Here's the drawing with two shaded views (mm, measured from the low corner). I have some questions. Give positions to 0.01 mm unless a question says otherwise; leave off trailing zeros. Write each loop counter-clockwise with the first axis right and the second up, starting at its lowest first coordinate (ties: lowest second). Pieces come first, ordered by that corner, then holes. Notation, with made-up numbers: M 75,89.5 L 128,89.5 A28 ccw 128,117.5 Z; hole C 43,-32 d9. An arc over 180 degrees is marked long. Answer as CSV lines item,"result". Start each with the question number.
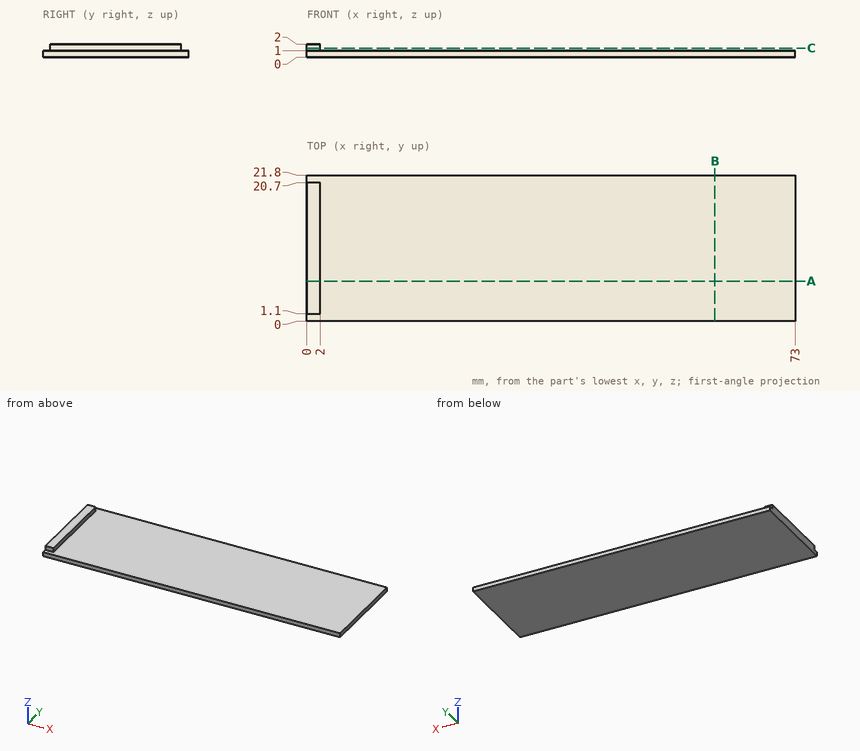
1. Will these pins go through, and if not, where does the flat tip stop? P1, Ø0.8, axis at x = 1, z = 1.5, coming from the +Y side; P2, Ø2, axis at x = 63.5, y = 12, coming from the +Z side; P3, Ø0.5, axis at y = 10.5, z = 1.5, coming from the +X side.
2. Imagine slicing it at C-C, the plane z = 1.4. Please give me the cut outline in (x, y).
3. Please list where these lines run through material, in increasing order: line 1 (X direction, y = 8.5, z = 1.6); line 2 (Z direction, x = 39, y = 4.5).
4. Imagine slicing it at A-A, the plane y = 6. Please give me the cut outline in (x, z), plus the area to 3 significant figures.
5. Imagine slicing it at B-B, the plane x = 61. Please give me the cut outline in (y, z), plus the area to 3 significant figures.
Solutions:
1,P1,"y = 20.7"
1,P2,"z = 1"
1,P3,"x = 2"
2,outline,"M 0,1.1 L 2,1.1 L 2,20.7 L 0,20.7 Z"
3,line 1,"0 to 2"
3,line 2,"0 to 1"
4,outline,"M 0,0 L 73,0 L 73,1 L 2,1 L 2,2 L 0,2 Z"
4,area,"75.0 mm²"
5,outline,"M 0,0 L 21.8,0 L 21.8,1 L 0,1 Z"
5,area,"21.8 mm²"
